Input: part model. Units: mm. Frame: model coordinates. A direction names the side the tool comes from. Coordinates: 2 decimals unless noted, no trailing zeros. Order: outer loops, then holes, each group sorted by start corner. A loop starts at its lowest first (then second) coordinate and runs counter-clockwise, first axis right, second up. Notation, with made-up numbers: (12.5, 21) -> (59.5, 21) arc R22 cw to (59.5, 32) -> close; hole circle Ø5 at (-10, 61.5). An arc over 180 degrees is marked (long way). Answer as CSV lines item,"result".
from build123d import *

# Parameters (mm, degrees)
CUT_EXTRUDE1_DEPTH = 15.976868681
SCALE1_SCALE       = 5.55


with BuildPart() as part:
    # Sketch1 → Base-Revolve (revolve)
    with BuildSketch(Plane.XY):
        with BuildLine():
            Line((0, 17.399), (0, -17.399))
            Line((0, -17.399), (18.415, -17.399))
            ThreePointArc((18.415, -17.399), (19.460122177, 0.417396993), (13.97, 17.399))
            Line((13.97, 17.399), (0, 17.399))
        make_face()
    revolve(axis=Axis((0, 64.099865047, 0), (0, -1, 0)))

    # Sketch2 → Cut-Extrude1 (cut, symmetric)
    with BuildSketch(Plane(origin=(0, 0, 0), x_dir=(0, 0, -1), z_dir=(1, 0, 0))):
        Polygon((-13.944000247, -17.399), (-19.286363897, 1.651), (-22.841821799, 1.651), (-22.841821799, -17.894237605), (-13.944000247, -17.894237605), align=None)
        Polygon((19.796019511, -3.429), (22.737840025, -3.429), (22.737840025, -17.894237605), (14.094585635, -17.894237605), (14.094585635, -17.399), align=None)
    extrude(amount=CUT_EXTRUDE1_DEPTH, both=True, mode=Mode.SUBTRACT)

    # Sketch3 → Boss-Revolve1 (revolve)
    with BuildSketch(Plane.XY):
        with BuildLine():
            Line((0, 36.703), (0, 11.303))
            ThreePointArc((0, 11.303), (12.7, 24.003), (0, 36.703))
        make_face()
    revolve(axis=Axis((0, 0, 0), (0, 1, 0)))

    # Sketch5 → Boss-Revolve2 (revolve)
    with BuildSketch(Plane.XY):
        with BuildLine():
            Line((10.922, -16.2306), (10.922, -32.7914))
            ThreePointArc((10.922, -32.7914), (19.2024, -24.511), (10.922, -16.2306))
        make_face()
    boss_revolve2 = revolve(axis=Axis((10.922, -36.241550195, 0), (0, 1, 0)))

    # Mirror1: Boss-Revolve2 across plane
    add(boss_revolve2.mirror(Plane(origin=(0, 0, 0), x_dir=(0, 0, 1), z_dir=(1, 0, 0))))


with BuildPart() as part_1:
    # Scale1: scaled about (-1.79e-07, 0.806776092, -0.114453365)
    add(part.part.scale(SCALE1_SCALE).moved(Location((8.14e-07, -3.670831219, 0.520762811))))


solid = part_1.part
1. Contact query for flat-ended pins moving along their axis: pin 1 (12 mm diameter, centred on x = -55, z = 1, fed in from +Y); pin 2 (8 mm diameter, centred on x = -83.5, y = -45.5, fed in from +Z); pin 3 (3 mm diameter, centred on y = 88.5, z = -41, fed in from +X). Output: stop coordinate, or through.
Findings:
pin 1,"stops at y = 180.21"
pin 2,"stops at z = 76.51"
pin 3,"stops at x = 69.5"
2. Mould query, pull axis Y, two halves, no side actions, for faces 1 (the face through (1, -100.235, 1)), 2 (the face through (-0.94, -59.857, 89.234)). Classes: released by +Y, released by -Y, zero draft, split by the parting line, or undercut.
Findings:
face 1,"undercut"
face 2,"released by -Y"
3. Reachability of faces 3 (the face through (40, 92.894, -45)), 4 (the face through (0.9, -70.6, -89.8)) from +Z, -Z, +X, -X, +Y, -Y: full face, straight path, thin tool, end or side. Return the list, or none.
Findings:
face 3,"none"
face 4,"-Z, +X, -X, -Y"
4. Ray query, line 1 along Y through (x, z) = (62, 0); line 2 along Y through (x, z) = (31.5, 67); line 3 along Y through (x, z) = (44.5, 49.5). Return the intervals inside material, ascending.
Findings:
line 1,"y = -185.64 to 92.89, 96.02 to 163.07"
line 2,"y = -100.24 to 92.89"
line 3,"y = -100.24 to 92.89, 105.28 to 153.81"
5. Cut plane C-C (y = 107). Return the cut outline in (x, z).
Findings:
outline,"circle Ø133.56 at (0, 0.52)"
6. Cut plane B-B (y = 148). Return the cut outline in (x, z).
Findings:
outline,"circle Ø136.05 at (0, 0.52)"
7. Cut plane A-A (z = -41). State how many separate pieces and enclosed holes the cut face has, plus the area to 3 significant figures.
Findings:
separate pieces,"3"
enclosed holes,"0"
area,"47,500 mm2"
